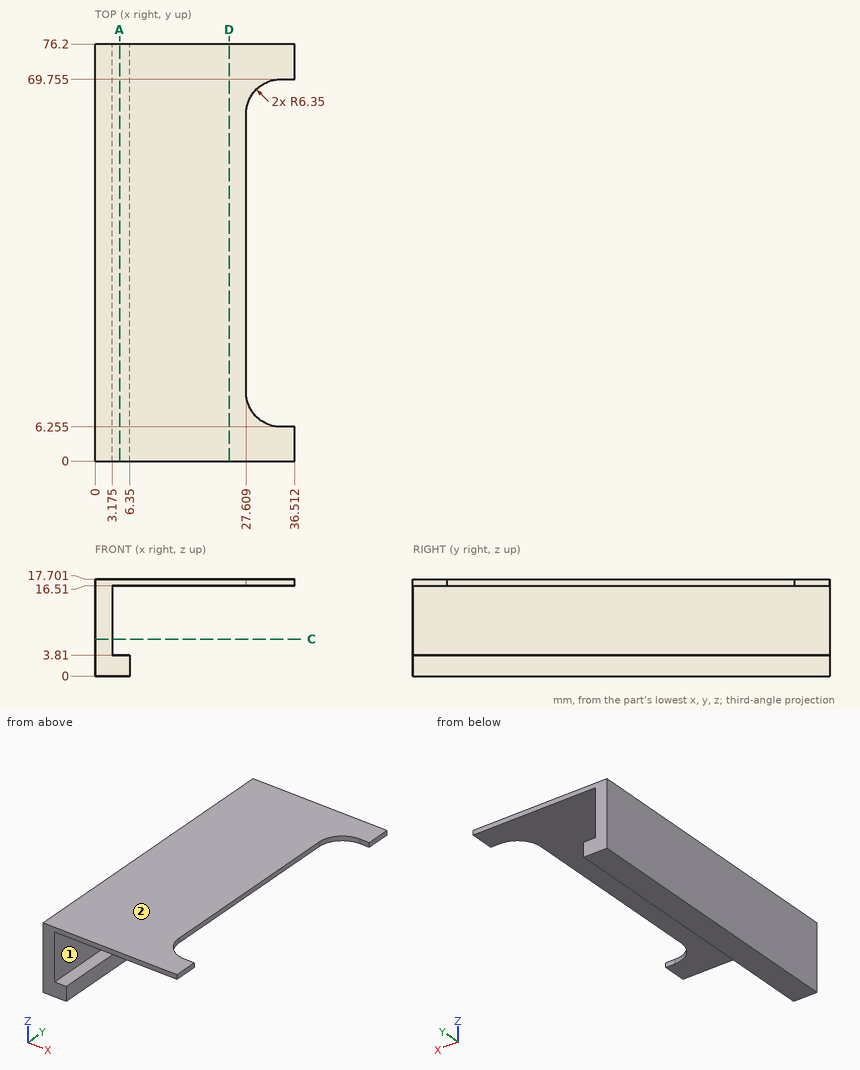
Source: three-view drawing plus pictorial views. Frame: mm from the lowest corner of the part. A direction names the side the tool comes from. Round coordinates to 2 decimals unless told otherwise and drop trailing zeros. Loops run counter-clockwise (first coordinate to the right, second up) from the corner with the lowest first, then second, coordinate; pieces in that order, holes last.
1. Access query for the marked faces 1 and 2. Directions: +Z, -Z, +X, -X, +Y, -Y. A direction counts if a zero-diameter tool reaches every point of the face in a straight line with its end or side. Return the directions, or none.
2. Section query A-A on x = 4.5. Output: boundary loops of the cut face in (y, z).
3. Section query D-D on x = 24.5. Output: boundary loops of the cut face in (y, z).
4. Contact query for flat-ended pins moving along their axis: pin 1 (4 mm diameter, centred on y = 41.5, z = 15, fed in from +X); pin 2 (16.5 mm diameter, centred on x = 24, y = 20.5, fed in from -Z); pin 3 (3 mm diameter, centred on y = 35, z = 2.5, fed in from +X). Output: stop coordinate, or through.
5. Section query C-C on z = 6.75. Output: boundary loops of the cut face in (x, y) (1 decimal), and give its area (3 significant figures).
6. Ray query, L1, parallel to X at y = 56.5, z = 9.5 (1 decimal); L2, parallel to Z at x = 27.5, y = 55. Return the intervals inside material, ascending.
Answers below:
1. face 1: +X, +Y, -Y
1. face 2: +Z, +X, -X, +Y, -Y
2. outline: (0, 0) - (76.2, 0) - (76.2, 3.81) - (0, 3.81) - close; (0, 16.51) - (76.2, 16.51) - (76.2, 17.7) - (0, 17.7) - close
3. outline: (0, 16.51) - (76.2, 16.51) - (76.2, 17.7) - (0, 17.7) - close
4. pin 1: stops at x = 27.61
4. pin 2: stops at z = 16.51
4. pin 3: stops at x = 6.35
5. outline: (0, 0) - (3.2, 0) - (3.2, 76.2) - (0, 76.2) - close
5. area: 242 mm2
6. L1: x = 0 to 3.2
6. L2: z = 16.51 to 17.7
